The model under review builds one solid part; all positions refer to its coordinate system, in mm. Face numbers are marked on the shaded views. A direction names the side the tool comes from. Round coordinates to 2 decimals unless told otherwise and drop trailing zeros. Order: outer loops, then holes, each group sorted by start corner. A loop starts at its lowest first (then second) coordinate and runs counter-clockwise, first axis right, second up.
1) Machinability: for the marked faces 1, 2 and 3, which of the approach directions +Z, -Z, +X, -X, +Y, -Y give a long, thin tool a straight path to every point of the face, cutting with its end or side? Answer none if there is none.
2) Consider section C-C (y = 10). Give the boundary of the cut face in (x, z), then the cut area to 3 significant figures.
3) Clearance check with flat-ended pins moving along their axes: P1, Ø1, axis at y = 6.5, z = 7, coming from the +X side; P2, Ø6, axis at y = 13.5, z = -4.5, coming from the +X side; P3, Ø3, axis at x = -1.5, y = 20, coming from the +Z side. State where each tip first meets the part, or that it passes through.
4) Consider section B-B (x = 2). Give the boundary of the cut face in (y, z), then the cut area to 3 significant figures.
5) Consider section A-A (z = 0). Give the boundary of the cut face in (x, y), then the cut area to 3 significant figures.
6) To check wall thickness, follow L1, parallel to Y at x = -4, z = 7.5; L2, parallel to Y at x = -0.5, z = 4.75; L3, parallel to Z at x = -0.25, y = 33. State the ranges of each line that lie inside material, in increasing order.
7) Consider section D-D (y = 19). Give the boundary of the cut face in (x, z), then the cut area to 3 significant figures.
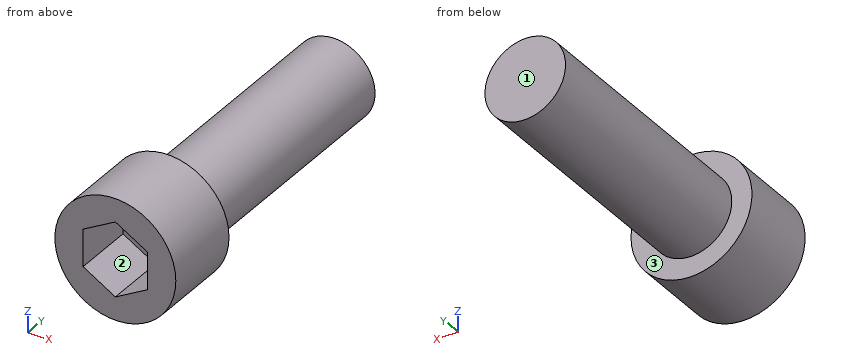
from build123d import *

# Parameters (mm, degrees)
F0_R     = 9
F1_DEPTH = 12
F2_R     = 6
F3_DEPTH = 37.5
F5_DEPTH = 9


with BuildPart() as f1:
    # F0 (on Front) → F1 (new body)
    with BuildSketch(Plane.XZ):
        Circle(F0_R)
    extrude(amount=-F1_DEPTH)

    # F2 (on face) → F3 (join)
    with BuildSketch(Plane(origin=(0, 12, 0), x_dir=(-1, 0, 0), z_dir=(0, 1, 0))):
        Circle(F2_R)
    extrude(amount=F3_DEPTH)

    # F4 (on face) → F5 (cut)
    with BuildSketch(Plane.XZ):
        Polygon((4.8, -2.771281), (4.8, 2.771281), (0, 5.542563), (-4.8, 2.771281), (-4.8, -2.771281), (0, -5.542563), align=None)
    extrude(amount=-F5_DEPTH, mode=Mode.SUBTRACT)


solid = f1.part
Answer below:
1. face 1: +Z, -Z, +X, -X, +Y
1. face 2: -Y
1. face 3: +Y
2. outline: circle Ø18 at (0, 0)
2. area: 254 mm2
3. P1: stops at x = 6.22
3. P2: stops at x = 8.8
3. P3: stops at z = 6
4. outline: (0, -8.77) - (12, -8.77) - (12, -5.66) - (49.5, -5.66) - (49.5, 5.66) - (12, 5.66) - (12, 8.77) - (0, 8.77) - (0, 4.39) - (9, 4.39) - (9, -4.39) - (0, -4.39) - close
4. area: 556 mm2
5. outline: (-9, 0) - (-4.8, 0) - (-4.8, 9) - (4.8, 9) - (4.8, 0) - (9, 0) - (9, 12) - (6, 12) - (6, 49.5) - (-6, 49.5) - (-6, 12) - (-9, 12) - close
5. area: 580 mm2
6. L1: y = 0 to 12
6. L2: y = 9 to 49.5
6. L3: z = -5.99 to 5.99
7. outline: circle Ø12 at (0, 0)
7. area: 113 mm2
